from build123d import *

# Parameters (mm, degrees)
F0_R      = 12.7
F1_DEPTH  = 6.35
F2_R      = 9.525
F3_DEPTH  = 12.7
F4_R      = 12.7
F5_DEPTH  = 6.35
F6_R      = 1.6002
F7_R      = 1.1938
F8_DEPTH  = 3.175
F9_R      = 6.35
F10_DEPTH = 25.401


with BuildPart() as f1:
    # F0 (on Front) → F1 (new body)
    with BuildSketch(Plane.XZ):
        Circle(F0_R)
    extrude(amount=F1_DEPTH)

    # F2 (on face) → F3 (join)
    with BuildSketch(Plane.XZ.offset(6.35)):
        Circle(F2_R)
    extrude(amount=F3_DEPTH)

    # F4 (on face) → F5 (join)
    with BuildSketch(Plane.XZ.offset(19.05)):
        Circle(F4_R)
    extrude(amount=F5_DEPTH)

    # F6
    f6_edges = [f1.edges().sort_by_distance(p)[0] for p in [
        (-12.7, -25.4, 0),
        (-12.7, -19.05, 0),
        (-12.7, -6.35, 0),
        (-12.7, 0, 0),
    ]]
    fillet(f6_edges, radius=F6_R)

    # F7 (on face) → F8 (cut)
    with BuildSketch(Plane.XZ.offset(25.4)):
        with Locations((-8.255, 0)):
            Circle(F7_R)
        with Locations((0, -8.255)):
            Circle(F7_R)
        with Locations((8.255, 0)):
            Circle(F7_R)
        with Locations((0, 8.255)):
            Circle(F7_R)
    extrude(amount=-F8_DEPTH, mode=Mode.SUBTRACT)

    # F9 (on face) → F10 (cut, through all)
    with BuildSketch(Plane.XZ.offset(25.4)):
        Circle(F9_R)
    extrude(amount=-F10_DEPTH, mode=Mode.SUBTRACT)


solid = f1.part
Design review of the part built by this model. Coordinates are the model's own, in mm. A direction names the side the tool comes from. Give positions to 0.01 mm unless a question says otherwise; leave off trailing zeros. Write each loop counter-clockwise with the first axis right and the second up, starting at its lowest first coordinate (ties: lowest second). Pieces come first, ordered by that corner, then holes. Notation, with made-up numbers: M 78.25,-22.75 L 93.25,-22.75 A16 ccw 93.25,2.25 Z; hole C 54,-31 d9. An arc over 180 degrees is marked long. Answer as a JSON object with one key per item and string values. Group by question number.
1) We need section C-C (y = -4). Give the boundary of the cut face in (x, z).
2) Tool access review of faces 4 (the face through (-2.75, -3.15, -12.4)), 5 (the face through (8, -22.225, 0)), 6 (the face through (-5, -6.35, 8.3)): name each direction out of +Z, -Z, +X, -X, +Y, -Y from which nothing blocks a thin tool from reaching the whole face with its end or side.
3) Mouldability with a two-part tool opening along X and no side actions: class faces 1 (the face through (-7.559, -12.611, -5.796)), 2 (the face through (0, -22.225, 8)), 3 (the face through (5, -25.4, -5)) as released by +X, released by -X, zero draft, split by the parting line, or undercut.
4) Clearance check with flat-ended pins moving along their axes: pin 1 Ø12 at (x, y) = (-5, -14.5) entering from +Z; pin 2 Ø0.7 at (x, z) = (-9, 0) entering from -Y (3 decimals); pin 3 Ø4 at (x, y) = (-9.5, -2.5) entering from +Z. State where each tip first meets the part, or that it passes through.
5) For line 1 along Z through (x, y) = (0, -23.85); line 2 along Z through (x, y) = (0, -24.3); line 3 along Y through (x, z) = (9.75, 5.25), list the stretches that pass through material, from the lowest coordinate up.
Answer key:
{
 "1": {"outline": "C 0,0 d25.4; hole C 0,0 d12.7"},
 "2": {"face 4": "+Y, -Y", "face 5": "-Y", "face 6": "none"},
 "3": {"face 1": "split by the parting line", "face 2": "undercut", "face 3": "zero draft"},
 "4": {"pin 1": "stops at z = 12.29", "pin 2": "stops at y = -22.225", "pin 3": "stops at z = 10.25"},
 "5": {"line 1": "z = -12.7 to -9.45, -7.06 to -6.35, 6.35 to 7.06, 9.45 to 12.7", "line 2": "z = -12.62 to -9.45, -7.06 to -6.35, 6.35 to 7.06, 9.45 to 12.62", "line 3": "y = -25.4 to -19.05, -6.35 to 0"}
}
